Source: three-view drawing plus pictorial views. Frame: mm from the lowest corner of the part. A direction names the side the tool comes from. Round coordinates to 2 decimals unless told otherwise and drop trailing zeros. Order: outer loops, then holes, each group sorted by start corner. A loop starts at its lowest first (then second) coordinate and runs counter-clockwise, first axis right, second up. Notation, with made-up numbers: M -39,58 L 1,58 A27 cw 1,81 Z; hole C -30,58 d2. An arc over 180 degrees is marked long. Return JSON: item names as keys, results as strings. Group by question number.
Q1. Cut plane D-D on x = 15.5. Output: boundary loops of the cut face in (y, z), and give its area (3 significant figures).
Q2. Ray query, probe 1 along X at (y, z) = (10.8, 22.25); probe 2 along X at (y, z) = (6.25, 38.5); probe 3 along X at (y, z) = (10.6, 10.2). Return the intervals inside material, ascending.
Q3. Cut plane C-C on z = 32.05. Output: boundary loops of the cut face in (x, y), and give its area (3 significant figures).
Q4. Access query for the marked faces 1, 2 and 3. Directions: +Z, -Z, +X, -X, +Y, -Y. A direction counts if a zero-diameter tool reaches every point of the face in a straight line with its end or side. Return the directions, or none.
Q5. Cut plane A-A on x = 28.5. Output: boundary loops of the cut face in (y, z), and give its area (3 significant figures).
Q6. Contact query for flat-ended pins moving along their axis: pin 1 (4 mm diameter, centred on x = 38, z = 26, fed in from -Y); pin 2 (1.5 mm diameter, centred on x = 58.5, z = 40.5, fed in from -Y); pin 3 (2 mm diameter, centred on x = 57.5, z = 20, fed in from -Y). Output: stop coordinate, or through.
Q7. Cut plane B-B on y = 1.5. Output: boundary loops of the cut face in (x, z).
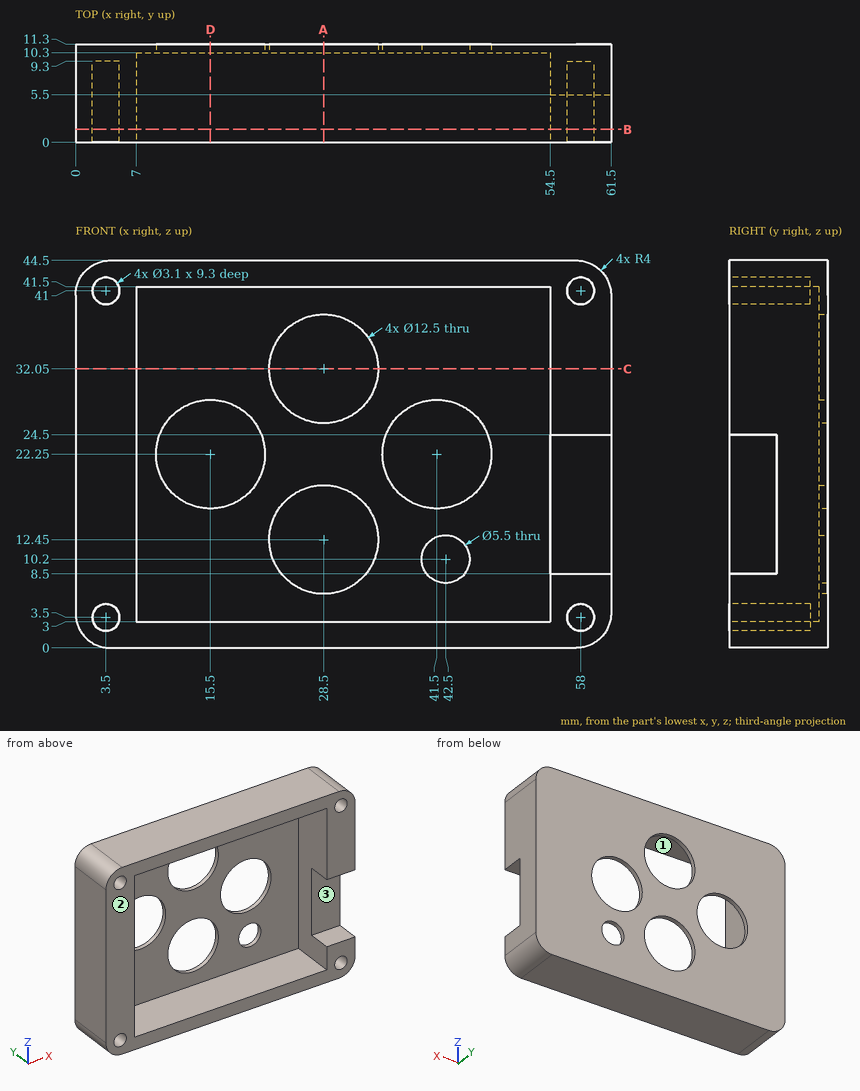
Result sheet:
{
 "1": {"outline": "M 0,0 L 11.3,0 L 11.3,16 L 10.3,16 L 10.3,3 L 0,3 Z; M 0,41.5 L 10.3,41.5 L 10.3,28.5 L 11.3,28.5 L 11.3,44.5 L 0,44.5 Z", "area": "93.8 mm²"},
 "2": {"probe 1": "x = 0 to 9.25, 21.75 to 35.25, 47.75 to 61.5", "probe 2": "x = 0 to 7, 54.5 to 61.5", "probe 3": "x = 0 to 22.67, 34.33 to 39.75, 45.25 to 61.5"},
 "3": {"outline": "M 0,0 L 7,0 L 7,10.3 L 22.25,10.3 L 22.25,11.3 L 0,11.3 Z; M 34.75,10.3 L 54.5,10.3 L 54.5,0 L 61.5,0 L 61.5,11.3 L 34.75,11.3 Z", "area": "193 mm²"},
 "4": {"face 1": "-Y", "face 2": "+Z, -Z, +X, -X, -Y", "face 3": "+X, -Y"},
 "5": {"outline": "M 0,0 L 11.3,0 L 11.3,6.2 L 10.3,6.2 L 10.3,3 L 0,3 Z; M 0,41.5 L 10.3,41.5 L 10.3,38.3 L 11.3,38.3 L 11.3,44.5 L 0,44.5 Z; M 10.3,18.7 L 11.3,18.7 L 11.3,25.8 L 10.3,25.8 Z", "area": "81.3 mm²"},
 "6": {"pin 1": "stops at y = 10.3", "pin 2": "stops at y = 9.3", "pin 3": "stops at y = 5.5"},
 "7": {"outline": "M 0,4 A4 ccw 4,0 L 57.5,0 A4 ccw 61.5,4 L 61.5,8.5 L 54.5,8.5 L 54.5,3 L 7,3 L 7,41.5 L 54.5,41.5 L 54.5,24.5 L 61.5,24.5 L 61.5,40.5 A4 ccw 57.5,44.5 L 4,44.5 A4 ccw 0,40.5 Z; hole C 3.5,3.5 d3.1; hole C 3.5,41 d3.1; hole C 58,3.5 d3.1; hole C 58,41 d3.1"}
}
